The model under review builds one solid part; all positions refer to its coordinate system, in mm. Face numbers are marked on the shaded views. A direction names the side the tool comes from. Coordinates: 2 decimals unless noted, no trailing zeros. Write each loop counter-clockwise with the first axis right and the second up, starting at its lowest first coordinate (ties: lowest second). Pieces come first, ordered by that corner, then holes. Notation, with made-up numbers: (76, 0.25) - (125, 0.25) arc R4 cw to (125, 4.25) - close; hole circle Ø7 at (77, 60.25). An arc over 180 degrees is marked (long way). Return JSON: item names as keys, results as strings. Group by question number.
(1) To check wall thickness, follow L1, parallel to X at y = 23, z = 11; L2, parallel to Y at x = 33.5, z = 34; L3, parallel to Z at x = 43, y = 5.5. State the ranges of each line that lie inside material, in increasing order. Write a range as from..to.
(2) We need section D-D on x = 15. State the section outline as (y, z) points, then the cut area to 3 significant figures.
(3) Tool access review of the marked faces 5 and 6: name each direction out of +Z, -Z, +X, -X, +Y, -Y from which nothing blocks a thin tool from reaching the whole face with its end or side.
(4) We need section A-A on z = 22. State the section outline as (x, y) points, then the cut area to 3 significant figures.
(5) For pin 1 Ø6 at (x, z) = (12, 8.5) entering from +Y; pin 2 Ø21 at (x, y) = (16.5, 18.5) entering from -Z, all flat-tipped, find the tip position at first contact; note any pin that passes through.
(6) Draft analysis for pull direction X (two halves, no side actions). For the marked faces 1, 2, 3 and 4, state which applies: released by +X, released by -X, zero draft, split by the parting line, or undercut.
(7) We need section C-C on z = 48. State the section outline as (x, y) points, then the cut area to 3 significant figures.
(8) We need section B-B on y = 23.5. State the section outline as (x, z) points.
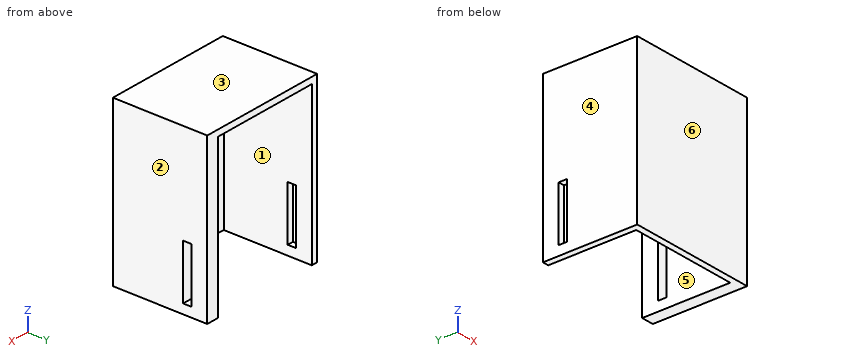
Autodesk Inventor part; units mm, degrees
ref_plane "YZ Plane" through (0, 0, 0) normal (1, 0, 0) x (0, 1, 0)
ref_plane "XZ Plane" through (0, 0, 0) normal (0, 1, 0) x (-1, 0, 0)
ref_plane "XY Plane" through (0, 0, 0) normal (0, 0, 1) x (1, 0, 0)
sketch "Sketch2" plane through (0, 0, 0) normal (0, 1, 0) x (-1, 0, 0)
  line L0 (0, 0) -> (-59, 0)
  line L1 (-59, 0) -> (-59, 78)
  line L2 (-59, 78) -> (0, 78)
  line L3 (0, 78) -> (0, 0)
  dimension "d0" = 59
  dimension "d1" = 78
extrude "Extrusion1" add sketch "Sketch2" along normal blind 45
shell "Shell1" thickness 3 removed faces 1 at (39.3333, 45, 52)
sketch "Sketch4" plane through (59, 0, 0) normal (0, 0, -1) x (-1, 0, 0)
  point P0 (59, 0)
sketch "Sketch5" plane through (3, 3, 3) normal (0, 0, 1) x (1, 0, 0)
  line L0 (0, 0) -> (0, 42)
  line L1 (0, 42) -> (53, 42)
  line L2 (0, 0) -> (53, 0)
  line L3 (53, 0) -> (53, 42)
  line L4 (53, 42) -> (0, 42)
  line L5 (0, 42) -> (0, 0)
  point P0 (-3, -3)
extrude "Extrusion3" cut sketch "Sketch5" against normal blind 10
sketch "Sketch6" plane through (0, 0, 0) normal (-1, 0, 0) x (0, 0, 1)
  line L0 (4.5, 37.5) -> (30.5, 37.5)
  line L1 (30.5, 37.5) -> (30.5, 33.5)
  line L2 (30.5, 33.5) -> (4.5, 33.5)
  line L3 (4.5, 33.5) -> (4.5, 37.5)
  line L4 (0, 0) -> (0, 45)
  line L5 (0, 0) -> (78, 0)
  dimension "d19" = 26
  dimension "d20" = 4
  dimension "d21" = 4.5
  dimension "d22" = 33.5
sketch "Sketch7" plane through (59, 0, 78) normal (1, 0, 0) x (0, 0, -1)
  line L0 (0, 0) -> (78, 0)
  line L1 (0, 45) -> (78, 45)
  line L2 (78, 45) -> (78, 0)
  line L3 (78, 0) -> (0, 0)
  line L4 (0, 0) -> (0, 45)
extrude "Extrusion5" add sketch "Sketch7" along normal blind 3
extrude "Extrusion6" cut sketch "Sketch6" against normal through all
properties part number "arduino with shield box v04"
Ans:
{
 "1": {"L1": "0..3, 56..62", "L2": "0..3", "L3": "75..78"},
 "2": {"outline": "(0, 0) - (3, 0) - (3, 75) - (45, 75) - (45, 78) - (0, 78) - close", "area": "360 mm²"},
 "3": {"face 5": "-Z, +Y", "face 6": "+Z, -Z, +X, -X, -Y"},
 "4": {"outline": "(0, 0) - (62, 0) - (62, 33.5) - (56, 33.5) - (56, 3) - (3, 3) - (3, 33.5) - (0, 33.5) - close; (0, 37.5) - (3, 37.5) - (3, 45) - (0, 45) - close; (56, 37.5) - (62, 37.5) - (62, 45) - (56, 45) - close", "area": "528 mm²"},
 "5": {"pin 1": "y = 3", "pin 2": "z = 75"},
 "6": {"face 1": "undercut", "face 2": "released by +X", "face 3": "zero draft", "face 4": "released by -X"},
 "7": {"outline": "(0, 0) - (62, 0) - (62, 45) - (56, 45) - (56, 3) - (3, 3) - (3, 45) - (0, 45) - close", "area": "564 mm²"},
 "8": {"outline": "(0, 0) - (3, 0) - (3, 75) - (56, 75) - (56, 0) - (62, 0) - (62, 78) - (0, 78) - close"}
}
